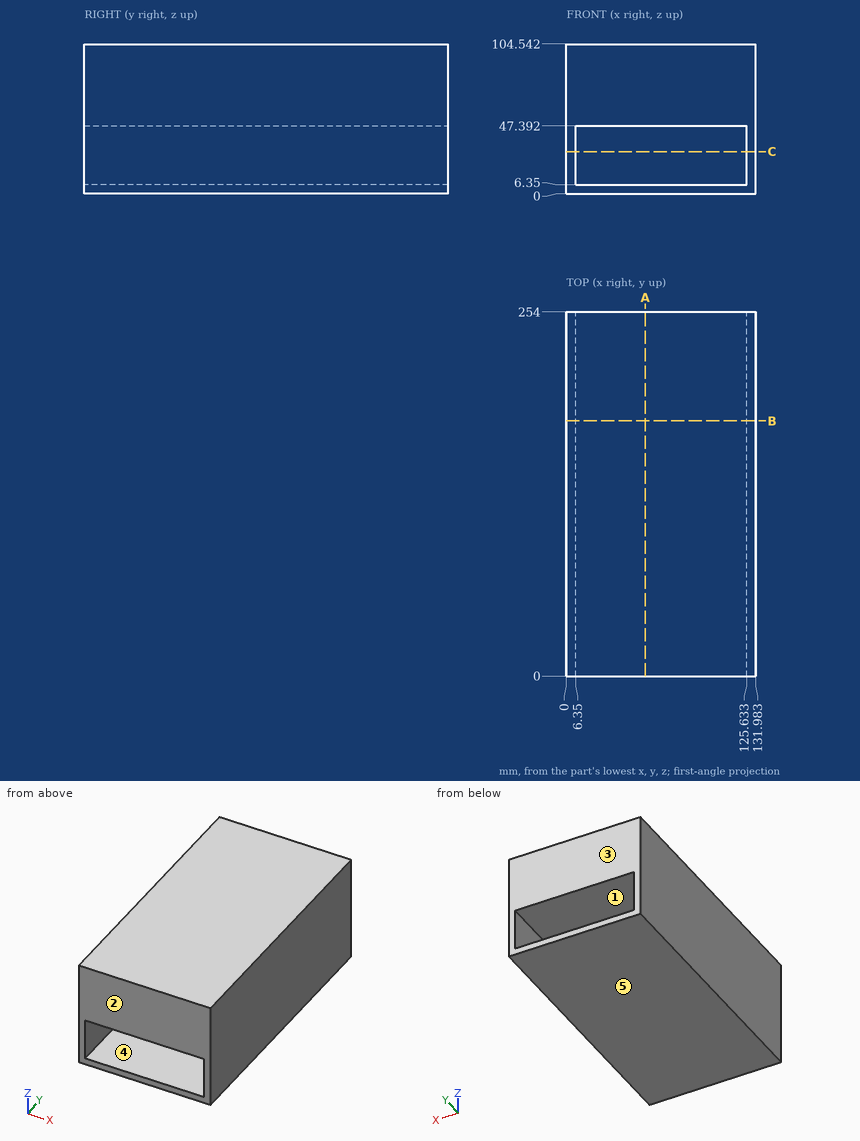
For this review, use the dimensioned drawing (mm, ordinates from the lowest corner) and the shaded views. A direction names the side the tool comes from. Give positions to 0.01 mm unless a question says otherwise; leave off trailing zeros. Order: outer loops, then holes, each group sorted by start corner. A loop starts at its lowest first (then second) coordinate and runs counter-clockwise, first axis right, second up. Notation, with made-up numbers: (74.5, 5.5) - (95.5, 5.5) arc R31 ccw to (95.5, 43.5) - close; hole circle Ø3 at (-12, 29.25). An arc over 180 degrees is marked (long way). Write item = value, one per line. Start each with the question number.
Q1. Mouldability with a two-part tool opening along Z and no side actions: class the marked faces 3, 4 and 5 as released by +Z, released by -Z, zero draft, split by the parting line, or undercut.
Q2. Clearance check with a flat-ended pin moving along its axis: pin 1 Ø12.5 at (y, z) = (121.5, 34.5) entering from -X. State where the tip first meets the part, or that it passes through.
Q3. We need section A-A on x = 55. State the section outline as (y, z) points.
Q4. We need section C-C on z = 29.5. State the section outline as (x, y) points.
Q5. We need section B-B on y = 178. State the section outline as (x, z) points.
Q6. To check wall thickness, follow L1, parallel to Z at x = 8, y = 30.5; L2, parallel to X at y = 62, z = 36.5. State the ranges of each line that lie inside material, in increasing order. Write a range as from..to.
Q7. Tool access review of the marked faces 1 and 2: name each direction out of +Z, -Z, +X, -X, +Y, -Y from which nothing blocks a thin tool from reaching the whole face with its end or side.
Working result:
q1.face_3 = zero draft
q1.face_4 = undercut
q1.face_5 = released by -Z
q2.pin_1 = 0
q3.outline = (0, 0) - (254, 0) - (254, 6.35) - (0, 6.35) - close; (0, 47.39) - (254, 47.39) - (254, 104.54) - (0, 104.54) - close
q4.outline = (0, 0) - (6.35, 0) - (6.35, 254) - (0, 254) - close; (125.63, 0) - (131.98, 0) - (131.98, 254) - (125.63, 254) - close
q5.outline = (0, 0) - (131.98, 0) - (131.98, 104.54) - (0, 104.54) - close; hole (6.35, 6.35) - (125.63, 6.35) - (125.63, 47.39) - (6.35, 47.39) - close
q6.L1 = 0..6.35, 47.39..104.54
q6.L2 = 0..6.35, 125.63..131.98
q7.face_1 = +Y, -Y
q7.face_2 = +Z, -Z, +X, -X, -Y
